The model under review builds one solid part; all positions refer to its coordinate system, in mm. A direction names the side the tool comes from. Round coordinates to 2 decimals unless told otherwise and drop trailing zeros. Order: outer loops, then holes, each group sorted by start corner. A loop starts at its lowest first (then second) coordinate and runs counter-clockwise, first axis right, second up. Notation, with made-up numbers: M -6,24 L 51,24 A23 cw 51,42 Z; hole C 23,18 d5. An arc over 180 degrees is marked long. Use a Markdown table: item, result. Add a question column.
1. The part is to be moulded in two halves that separate along X. For faces 3 (the flat face through (-38, 10, 2)), 4 (the cylindrical face through (-53.06, -0.8, 1.97)), 5 (the flat face through (-65, 0, 2)), say which applies: +X half, -X half, draft (parallel to the pull), parting line (faces both ways), or undercut.
2. To check wall thickness, follow probe 1 along Y at (x, z) = (0, 2.05); probe 2 along Y at (x, z) = (15, 2.3); probe 3 along Y at (x, z) = (55, 2.4). State the ranges of each line that lie inside material, in increasing order.
3. Consider section D-D on y = 0. State the section outline as (x, z) points, then the cut area to 3 significant figures.
4. Consider section B-B on y = 40. State the section outline as (x, z) points, then the cut area to 3 significant figures.
5. Insertion check: P1, Ø2, axis at y = 28, z = 1.5, coming from the +X side; P2, Ø2, axis at y = 37.5, z = 1.5, coming from the -X side; P3, Ø1.2, axis at x = 40, z = 2.5, coming from the +Y side. Each pin has a flat end and moves straight along its axis. Give the tip position at first contact, or say it passes through.
6. For faces 1 (the cylindrical face through (-37.1, 0.09, 1.97)), 2 (the flat face through (-10, 30, 2)), list the 3-axis set-ups (+Z, -Z, +X, -X, +Y, -Y) from which the entire face can be reached by the end or side of a thin tool; tool diameter is ignored.
7. Consider section A-A on x = 0. State the section outline as (y, z) points, then the cut area to 3 significant figures.
from build123d import *

# Parameters (mm, degrees)
SKETCH_1_W      = 130
SKETCH_1_H      = 20
SKETCH_1_R      = 2.1
SKETCH_1_W_2    = 20
SKETCH_1_H_2    = 40
EXTRUDE_1_DEPTH = 4
FILLET_1_R      = 3


with BuildPart() as part:
    # 草图1 → 凸台-拉伸1 (new body)
    # profile 1 of 2: a face of its own
    with BuildSketch(Plane.XY):
        Rectangle(SKETCH_1_W, SKETCH_1_H)
        with Locations((35, 0)):
            Circle(SKETCH_1_R, mode=Mode.SUBTRACT)
        with Locations((-35, 0)):
            Circle(SKETCH_1_R, mode=Mode.SUBTRACT)
        with Locations((-55, 0)):
            Circle(SKETCH_1_R, mode=Mode.SUBTRACT)
        with Locations((55, 0)):
            Circle(SKETCH_1_R, mode=Mode.SUBTRACT)
    # profile 2 of 2: a face of its own
    with BuildSketch(Plane.XY):
        with Locations((0, 30)):
            Rectangle(SKETCH_1_W_2, SKETCH_1_H_2)
        with Locations((0, 20)):
            Circle(SKETCH_1_R, mode=Mode.SUBTRACT)
        with Locations((0, 40)):
            Circle(SKETCH_1_R, mode=Mode.SUBTRACT)
    extrude(amount=EXTRUDE_1_DEPTH)

    # 圆角1
    fillet_1_edges = [part.edges().sort_by_distance(p)[0] for p in [
        (65, -10, 2),
        (-65, -10, 2),
        (-65, 10, 2),
        (-10, 10, 2),
        (-10, 50, 2),
        (10, 50, 2),
        (10, 10, 2),
        (65, 10, 2),
    ]]
    fillet(fillet_1_edges, radius=FILLET_1_R)


solid = part.part
Answer block:
| question | item | result |
|---|---|---|
| 1 | face 3 | draft |
| 1 | face 4 | undercut |
| 1 | face 5 | -X half |
| 2 | probe 1 | -10 to 17.9, 22.1 to 37.9, 42.1 to 50 |
| 2 | probe 2 | -10 to 10 |
| 2 | probe 3 | -10 to -2.1, 2.1 to 10 |
| 3 | outline | M -65,0 L -57.1,0 L -57.1,4 L -65,4 Z; M -52.9,0 L -37.1,0 L -37.1,4 L -52.9,4 Z; M -32.9,0 L 32.9,0 L 32.9,4 L -32.9,4 Z; M 37.1,0 L 52.9,0 L 52.9,4 L 37.1,4 Z; M 57.1,0 L 65,0 L 65,4 L 57.1,4 Z |
| 3 | area | 453 mm^2 |
| 4 | outline | M -10,0 L -2.1,0 L -2.1,4 L -10,4 Z; M 2.1,0 L 10,0 L 10,4 L 2.1,4 Z |
| 4 | area | 63.2 mm^2 |
| 5 | P1 | x = 10 |
| 5 | P2 | x = -10 |
| 5 | P3 | y = 10 |
| 6 | face 1 | +Z, -Z |
| 6 | face 2 | +Z, -Z, -X, +Y |
| 7 | outline | M -10,0 L 17.9,0 L 17.9,4 L -10,4 Z; M 22.1,0 L 37.9,0 L 37.9,4 L 22.1,4 Z; M 42.1,0 L 50,0 L 50,4 L 42.1,4 Z |
| 7 | area | 206 mm^2 |
